Here's how the part is built. I have some questions about the finished solid (model axes, mm). Round coordinates to 2 decimals unless told otherwise and drop trailing zeros. Loops run counter-clockwise (first coordinate to the right, second up) from the corner with the lowest first, then second, coordinate; pieces in that order, holes last. Notation, with made-up numbers: (38, 32.25) -> (78, 32.25) arc R32 cw to (78, 67.25) -> close; hole circle Ø6 at (13, -1). An arc over 180 degrees is marked (long way). Use one line per item in the form item = value. Start each with the question number.
Item 1: If I drill on L1, parallel to Y at x = 8, z = 27; L2, parallel to X at y = 26.5, z = -15.5; L3, parallel to X at y = 12, z = 3.5, over which ranges is the centre line in solid material (lowest first)? Write a range as [from, to].
Item 2: If we section it at D-D (z = -11): State how many separate pieces and enclosed holes the cut face has, then the cut area to 3 significant figures.
Item 3: Thinking about a two-plate mould opening in Z: for faces 1 (the face through (3.734, 38.454, 9.893)), 2 (the face through (1.52, 22.33, -18.13)), 3 (the face through (2, 0, 6)), which applies, released by +Z, released by -Z, zero draft, split by the parting line, or undercut?
Item 4: If we section it at B-B (y = 23): Write out the boundary of the cut face in (x, z).
Item 5: I'm going to push flat-ended pins straight in: pin 1 Ø3.5 at (y, z) = (71, -3) entering from -X; pin 2 Ø2 at (y, z) = (55, -19) entering from -X; pin 3 Ø12 at (y, z) = (53.5, -19.5) entering from +X; pin 4 Ø2 at (y, z) = (67.5, 31) entering from -X. Where does each tip first touch, or does it pass through?
Item 6: If we section it at C-C (z = 31): Write out the boundary of the cut face in (x, y), then the cut area to 3 significant figures.
Item 7: If we section it at A-A (y = 39): Write out the boundary of the cut face in (x, z), then the cut area to 3 significant figures.
```python
from build123d import *

# Parameters (mm, degrees)
EXTRUSION1_DEPTH = 78
EXTRUSION3_REACH = 32.949
ESQUISSE2_R      = 2
ESQUISSE2_W      = 25
ESQUISSE2_H      = 58
CONG_1_R         = 3
ESQUISSE3_R      = 1.1
EXTRUSION4_DEPTH = 3


with BuildPart() as part:
    # Esquisse1 → Extrusion1 (new body)
    with BuildSketch(Plane(origin=(0, 0, 0), x_dir=(1, 0, 0), z_dir=(0, 1, 0))):
        with BuildLine():
            Line((0, 0), (0, 30))
            Line((0, 30), (3, 30))
            Line((3, 30), (3, 0))
            ThreePointArc((3, 0), (4.257195182, -12.918344113), (7.981600437, -25.351885839))
            Line((7.981600437, -25.351885839), (15.549327553, -43.864840933))
            Line((15.549327553, -43.864840933), (12.772384289, -45))
            Line((12.772384289, -45), (5.204657173, -26.487044906))
            ThreePointArc((5.204657173, -26.487044906), (1.313487503, -13.496777432), (0, 0))
        make_face()
    extrude(amount=EXTRUSION1_DEPTH)

    # Esquisse2 → Extrusion3 (cut, up to next)
    with BuildSketch(Plane(origin=(-4.817679226, 0, 1.969371261), x_dir=(0.378386356, 0, 0.925647755), z_dir=(-0.925647755, 0, 0.378386356)), mode=Mode.PRIVATE) as extrusion3_sk1:
        with Locations((41.487044906, 5)):
            Circle(ESQUISSE2_R)
    extrusion3_tool1 = extrude(extrusion3_sk1.sketch, amount=-EXTRUSION3_REACH, mode=Mode.PRIVATE) & part.part
    add(extrusion3_tool1.solids().sort_by_distance((10.880453, 5, 40.371761))[0], mode=Mode.SUBTRACT)
    # Esquisse2 → Extrusion3 (cut, up to next)
    with BuildSketch(Plane(origin=(-4.817679226, 0, 1.969371261), x_dir=(0.378386356, 0, 0.925647755), z_dir=(-0.925647755, 0, 0.378386356)), mode=Mode.PRIVATE) as extrusion3_sk2:
        with Locations((41.487044906, 73)):
            Circle(ESQUISSE2_R)
    extrusion3_tool2 = extrude(extrusion3_sk2.sketch, amount=-EXTRUSION3_REACH, mode=Mode.PRIVATE) & part.part
    add(extrusion3_tool2.solids().sort_by_distance((10.880453, 73, 40.371761))[0], mode=Mode.SUBTRACT)
    # Esquisse2 → Extrusion3 (cut, up to next)
    with BuildSketch(Plane(origin=(-4.817679226, 0, 1.969371261), x_dir=(0.378386356, 0, 0.925647755), z_dir=(-0.925647755, 0, 0.378386356)), mode=Mode.PRIVATE) as extrusion3_sk3:
        with Locations((33.987044906, 39)):
            Rectangle(ESQUISSE2_W, ESQUISSE2_H)
    extrusion3_tool3 = extrude(extrusion3_sk3.sketch, amount=-EXTRUSION3_REACH, mode=Mode.PRIVATE) & part.part
    add(extrusion3_tool3.solids().sort_by_distance((8.042555, 39, 33.429403))[0], mode=Mode.SUBTRACT)

    # Congé1
    cong_1_edges = [part.edges().sort_by_distance(p)[0] for p in [
        (14.160855921, 78, 44.432420466),
        (14.160855921, 0, 44.432420466),
    ]]
    fillet(cong_1_edges, radius=CONG_1_R)

    # Esquisse3 → Extrusion4 (cut)
    with BuildSketch(Plane(origin=(3, 0, 0), x_dir=(0, 0, -1), z_dir=(1, 0, 0))):
        with Locations((3, 31)):
            Circle(ESQUISSE3_R)
        with Locations((11, 31)):
            Circle(ESQUISSE3_R)
        with Locations((19, 31)):
            Circle(ESQUISSE3_R)
        with Locations((3, 39)):
            Circle(ESQUISSE3_R)
        with Locations((19, 39)):
            Circle(ESQUISSE3_R)
        with Locations((19, 47)):
            Circle(ESQUISSE3_R)
        with Locations((11, 47)):
            Circle(ESQUISSE3_R)
        with Locations((3, 47)):
            Circle(ESQUISSE3_R)
        with Locations((3, 23)):
            Circle(ESQUISSE3_R)
        with Locations((11, 23)):
            Circle(ESQUISSE3_R)
        with Locations((19, 23)):
            Circle(ESQUISSE3_R)
        with Locations((3, 15)):
            Circle(ESQUISSE3_R)
        with Locations((11, 15)):
            Circle(ESQUISSE3_R)
        with Locations((19, 15)):
            Circle(ESQUISSE3_R)
        with Locations((3, 7)):
            Circle(ESQUISSE3_R)
        with Locations((11, 7)):
            Circle(ESQUISSE3_R)
        with Locations((19, 7)):
            Circle(ESQUISSE3_R)
        with Locations((3, 71)):
            Circle(ESQUISSE3_R)
        with Locations((3, 55)):
            Circle(ESQUISSE3_R)
        with Locations((3, 63)):
            Circle(ESQUISSE3_R)
        with Locations((11, 71)):
            Circle(ESQUISSE3_R)
        with Locations((11, 63)):
            Circle(ESQUISSE3_R)
        with Locations((11, 55)):
            Circle(ESQUISSE3_R)
        with Locations((19, 55)):
            Circle(ESQUISSE3_R)
        with Locations((19, 63)):
            Circle(ESQUISSE3_R)
        with Locations((19, 71)):
            Circle(ESQUISSE3_R)
    extrude(amount=-EXTRUSION4_DEPTH, mode=Mode.SUBTRACT)


solid = part.part
```
Values found:
q1.L1 = [0, 10], [68, 78]
q1.L2 = [0, 3]
q1.L3 = [0.09, 3.09]
q2.separate_pieces = 9
q2.enclosed_holes = 0
q2.area = 181 mm2
q3.face_1 = released by -Z
q3.face_2 = undercut
q3.face_3 = zero draft
q4.outline = (0, -30) -> (3, -30) -> (3, -20.1) -> (0, -20.1) -> close; (0, -17.9) -> (3, -17.9) -> (3, -12.1) -> (0, -12.1) -> close; (0, -9.9) -> (3, -9.9) -> (3, -4.1) -> (0, -4.1) -> close; (0, -1.9) -> (3, -1.9) -> (3, 0) arc R67 cw to (6.26, 20.65) -> (3.48, 21.79) arc R70 ccw to (0, 0) -> close
q5.pin_1 = 0
q5.pin_2 = through
q5.pin_3 = 3
q5.pin_4 = 6.7
q6.outline = (7.05, 0) -> (10.29, 0) -> (10.29, 10) -> (7.05, 10) -> close; (7.05, 68) -> (10.29, 68) -> (10.29, 78) -> (7.05, 78) -> close
q6.area = 64.8 mm2
q7.outline = (0, -30) -> (3, -30) -> (3, -20.1) -> (0, -20.1) -> close; (0, -17.9) -> (3, -17.9) -> (3, -4.1) -> (0, -4.1) -> close; (0, -1.9) -> (3, -1.9) -> (3, 0) arc R67 cw to (6.26, 20.65) -> (3.48, 21.79) arc R70 ccw to (0, 0) -> close
q7.area = 142 mm2
